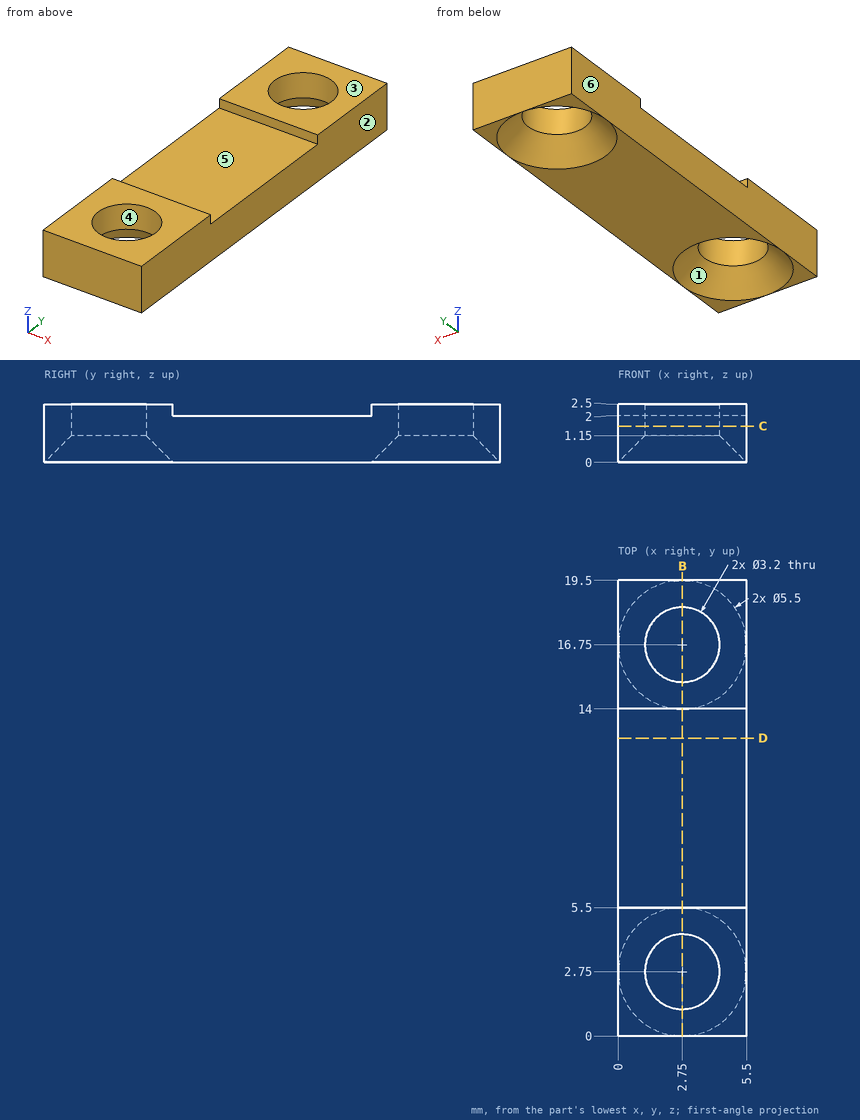
Job drawing, mm, ordinate dimensions from the low corner. One solid piece. A direction names the side the tool comes from. Coordinates: 2 decimals unless noted, no trailing zeros. Order: outer loops, then holes, each group sorted by start corner. A loop starts at its lowest first (then second) coordinate and runs counter-clockwise, first axis right, second up. Notation, with made-up numbers: (-23, 16.25) - (19, 16.25) arc R32 ccw to (19, 53.25) - close; hole circle Ø5 at (-8, 49). An arc over 180 degrees is marked (long way). Return JSON: item names as keys, results as strings. Group by question number.
1) Probe line 1 (Y direction, x = 2.75, z = 1.75); line 2 (Y direction, x = 1.75, z = 0.3); line 3 (Z direction, x = 1.15, y = 11.5). List the from-to ranges inside material, lowest first. Write a range as from..to.
2) Saw through at C-C, the plane z = 1.55. Write the cut outline in (x, y).
3) Mould opens along X. For the marked faces 1, 2, 3 and 4 say: released by +X, released by -X, zero draft, split by the parting line, or undercut.
4) Saw through at D-D, the plane y = 12.75. Write the cut outline in (x, z).
5) Saw through at B-B, the plane x = 2.75. Count the separate pieces of the cut face and the enclosed holes in it.
6) Tool access for the marked faces 5 and 6: list every direction of +Z, -Z, +X, -X, +Y, -Y with a clear straight run to the whole face (end or side of a thin tool).
Values found:
{
 "1": {"line 1": "y = 0..1.15, 4.35..15.15, 18.35..19.5", "line 2": "y = 0..0.51, 4.99..14.51, 18.99..19.5", "line 3": "z = 0..2"},
 "2": {"outline": "(0, 0) - (5.5, 0) - (5.5, 19.5) - (0, 19.5) - close; hole circle Ø3.2 at (2.75, 2.75); hole circle Ø3.2 at (2.75, 16.75)"},
 "3": {"face 1": "undercut", "face 2": "released by +X", "face 3": "zero draft", "face 4": "undercut"},
 "4": {"outline": "(0, 0) - (5.5, 0) - (5.5, 2) - (0, 2) - close"},
 "5": {"separate pieces": "3", "enclosed holes": "0"},
 "6": {"face 5": "+Z, +X, -X", "face 6": "+Z, -Z, -X, +Y, -Y"}
}
